```python
from build123d import *

# Parameters (mm, degrees)
SKETCH1_R           = 1.25
SKETCH1_R_2         = 1.175
BOSS_EXTRUDE1_DEPTH = 3.2
SKETCH2_R           = 0.5
BOSS_EXTRUDE2_DEPTH = 0.25
SKETCH3_W           = 2.907878402
SKETCH3_H           = 1.2
CUT_EXTRUDE1_DEPTH  = 1.7


with BuildPart() as part:
    # Sketch1 → Boss-Extrude1 (new body, symmetric)
    with BuildSketch(Plane.XY):
        with BuildLine():
            Line((-5.15, -3.3), (14.65, -3.3))
            Line((14.65, -3.3), (14.65, 6.9))
            Line((14.65, 6.9), (3.903939201, 7.7))
            Line((3.903939201, 7.7), (2.903939201, 7.7))
            ThreePointArc((2.903939201, 7.7), (1.95, 8.4), (0.996060799, 7.7))
            Line((0.996060799, 7.7), (-5.15, 7.7))
            Line((-5.15, 7.7), (-5.15, -3.3))
        make_face()
        Circle(SKETCH1_R, mode=Mode.SUBTRACT)
        with Locations((9.5, 0)):
            Circle(SKETCH1_R_2, mode=Mode.SUBTRACT)
    extrude(amount=BOSS_EXTRUDE1_DEPTH, both=True)

    # Sketch2 → Boss-Extrude2 (add, symmetric)
    with BuildSketch(Plane.XY):
        Polygon((-4.25, -3.3), (-1.45, -3.3), (-1.45, -10.3), (-2.15, -11), (-3.55, -11), (-4.25, -10.3), align=None)
        with Locations((-2.85, -9.5)):
            Circle(SKETCH2_R, mode=Mode.SUBTRACT)
        Polygon((3.35, -3.3), (6.15, -3.3), (6.15, -10.3), (5.45, -11), (4.05, -11), (3.35, -10.3), align=None)
        with Locations((4.75, -9.5)):
            Circle(SKETCH2_R, mode=Mode.SUBTRACT)
        Polygon((10.95, -3.3), (13.75, -3.3), (13.75, -10.3), (13.05, -11), (11.65, -11), (10.95, -10.3), align=None)
        with Locations((12.35, -9.5)):
            Circle(SKETCH2_R, mode=Mode.SUBTRACT)
    extrude(amount=BOSS_EXTRUDE2_DEPTH, both=True)

    # Sketch3 → Cut-Extrude1 (cut, through all)
    with BuildSketch(Plane(origin=(0, 7.7, 0), x_dir=(1, 0, 0), z_dir=(0, 1, 0))):
        with Locations((2.45, 2.6)):
            Rectangle(SKETCH3_W, SKETCH3_H)
        with Locations((2.45, -2.6)):
            Rectangle(SKETCH3_W, SKETCH3_H)
    extrude(amount=CUT_EXTRUDE1_DEPTH, mode=Mode.SUBTRACT)


solid = part.part
```
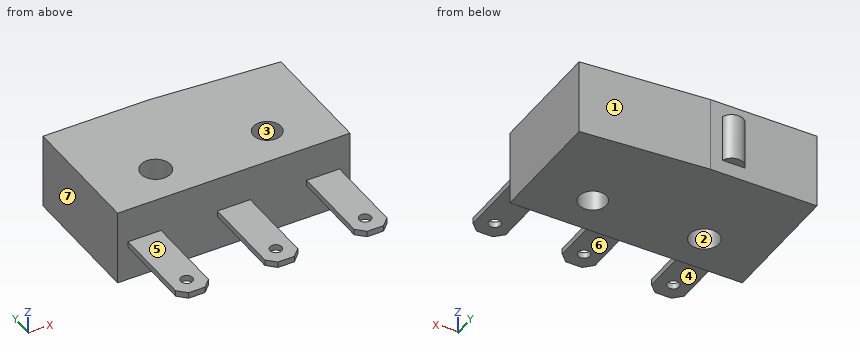
Source: CAD feature listing. Evaluate the final solid. Frame: model axes, mm. Face numbers are marked on the shaded views. A direction names the side the tool comes from. Coordinates: 2 decimals unless noted, no trailing zeros. Loops run counter-clockwise (first coordinate to the right, second up) from the corner with the lowest first, then second, coordinate; pieces in that order, holes last. Notation, with made-up numbers: (68.25, -11) -> (78.25, -11) arc R11 cw to (78.25, 0) -> close; hole circle Ø2 at (6, 39.5). An arc over 180 degrees is marked (long way). One line per item, written item: value. Start each with the question number.
Q1. Section query B-B, the plane y = -9.5. Return the cut outline in (x, z), and give its area (3 significant figures).
Q2. Mould query, pull axis Y, two halves, no side actions, for the marked faces 1, 2, 3 and 4. Classes: pulls with the +Y half, pulls with the -Y half, needs draft (parallel to the pull), parting line crosses it, or undercut.
Q3. Section query A-A, the plane x = 0. Return the cut outline in (y, z).
Q4. Set-up query: the marked faces 5, 6 and 7. Return all of +Z, -Z, +X, -X, +Y, -Y with unobstructed straight access to the full face (end or side cutting, diameter ignored); none if empty.
Q5. Line query: line 1 along Y through (x, z) = (-2.85, 0.1); line 2 along Y through (x, z) = (12.35, -0.05); line 3 along X through (y, z) = (0.75, 2.5). Output: solid intervals per line, ascending.
Q6. Section query D-D, the plane z = -1.5. Return the cut outline in (x, y) (3 decimals).
Q7. Contact query for flat-ended pins moving along their axis: P1, Ø0.8, axis at x = 12.5, y = -7.5, coming from the -Z side; P2, Ø0.6, axis at y = -8, z = 0, coming from the +X side; P3, Ø1.4, axis at x = 9.5, y = 0, coming from the +Z side; P4, Ø1.9, axis at x = -1.5, z = 0.5, coming from the +Y side. Output: stop coordinate, or through.
Q8. Section query C-C, the plane y = -5.25. Return the cut outline in (x, z).
Results:
1. outline: (-4.25, -0.25) -> (-3.35, -0.25) -> (-3.35, 0.25) -> (-4.25, 0.25) -> close; (-2.35, -0.25) -> (-1.45, -0.25) -> (-1.45, 0.25) -> (-2.35, 0.25) -> close; (3.35, -0.25) -> (4.25, -0.25) -> (4.25, 0.25) -> (3.35, 0.25) -> close; (5.25, -0.25) -> (6.15, -0.25) -> (6.15, 0.25) -> (5.25, 0.25) -> close; (10.95, -0.25) -> (11.85, -0.25) -> (11.85, 0.25) -> (10.95, 0.25) -> close; (12.85, -0.25) -> (13.75, -0.25) -> (13.75, 0.25) -> (12.85, 0.25) -> close
1. area: 2.70 mm^2
2. face 1: pulls with the +Y half
2. face 2: undercut
2. face 3: undercut
2. face 4: needs draft
3. outline: (-3.3, -3.2) -> (-1.25, -3.2) -> (-1.25, 3.2) -> (-3.3, 3.2) -> close; (1.25, -3.2) -> (7.7, -3.2) -> (7.7, 3.2) -> (1.25, 3.2) -> close
4. face 5: +Z, +X, -X, -Y
4. face 6: -Z, +X, -X, -Y
4. face 7: +Z, -Z, -X, +Y, -Y
5. line 1: -11 to -10, -9 to 7.7
5. line 2: -11 to -10, -9 to 7.07
5. line 3: -5.15 to -1, 1 to 8.6, 10.4 to 14.65
6. outline: (-5.15, -3.3) -> (14.65, -3.3) -> (14.65, 6.9) -> (3.904, 7.7) -> (2.904, 7.7) arc R1 ccw to (0.996, 7.7) -> (-5.15, 7.7) -> close; hole circle Ø2.5 at (0, 0); hole circle Ø2.35 at (9.5, 0)
7. P1: z = -0.25
7. P2: x = 13.75
7. P3: through
7. P4: y = 7.7
8. outline: (-4.25, -0.25) -> (-1.45, -0.25) -> (-1.45, 0.25) -> (-4.25, 0.25) -> close; (3.35, -0.25) -> (6.15, -0.25) -> (6.15, 0.25) -> (3.35, 0.25) -> close; (10.95, -0.25) -> (13.75, -0.25) -> (13.75, 0.25) -> (10.95, 0.25) -> close
